Design review of the part built by this model. Coordinates are the model's own, in mm. Face numbers are marked on the shaded views. A direction names the side the tool comes from. Coordinates: 2 decimals unless noted, no trailing zeros. Loops run counter-clockwise (first coordinate to the right, second up) from the corner with the lowest first, then second, coordinate; pieces in that order, holes last. Notation, with made-up numbers: (-13.5, 72) -> (34.5, 72) arc R20 cw to (34.5, 87) -> close; hole circle Ø5 at (83.5, -38). An arc over 180 degrees is marked (long way). Use one line per item in the form item = value. Start each with the question number.
1. Consider section C-C (x = 21). State the section outline as (y, z) points.
2. The part is to be moulded in two halves that separate along X. For the marked faces 1, 2 and 3, say which applies: released by +X, released by -X, zero draft, split by the parting line, or undercut.
3. For pin 1 (5 mm diameter, centred on x = -25, z = 7, fed in from +Y); pin 2 (4 mm diameter, centred on x = 11.5, z = 1.5, fed in from -Y); pin 3 (2 mm diameter, centred on x = 5.5, z = 8.5, fed in from +Y), all flat-tipped, find the tip position at first contact; note any pin that passes through.
4. Machinability: for the marked faces 4, 5 and 6, which of the approach directions +Z, -Z, +X, -X, +Y, -Y give a long, thin tool a straight path to every point of the face, cutting with its end or side? Answer none if there is none.
5. Wall thickness on line 1 (X direction, y = 2.4, z = 5); line 2 (Y direction, x = 24.5, z = 2.75); line 3 (X direction, y = 1.2, z = 5): over which ranges is each line inside the solid? List them lowest first. Write a range as from..to.
6. Consider section A-A (z = 5). State the section outline as (x, y) points.
7. Consider section D-D (y = 13). State the section outline as (x, z) points, then the cut area to 3 significant figures.
8. Consider section B-B (y = 4.75). State the section outline as (x, z) points, then the cut area to 3 significant figures.
from build123d import *

# Parameters (mm, degrees)
BOSS_EXTRUDE1_DEPTH = 10
SKETCH2_R           = 1.5875
CUT_EXTRUDE1_DEPTH  = 3.765696


with BuildPart() as part:
    # Sketch1 → Boss-Extrude1 (new body)
    with BuildSketch(Plane.XY):
        with BuildLine():
            Line((-20, 0), (-15, 0))
            ThreePointArc((-15, 0), (0, 15), (15, 0))
            Line((15, 0), (20, 0))
            Line((20, 0), (30, 0))
            Line((30, 0), (30, 3.765695973))
            Line((30, 3.765695973), (19.642289425, 3.765695973))
            ThreePointArc((19.642289425, 3.765695973), (0, 20), (-19.642289425, 3.765695973))
            Line((-19.642289425, 3.765695973), (-30, 3.765695973))
            Line((-30, 3.765695973), (-30, 0))
            Line((-30, 0), (-20, 0))
        make_face()
    extrude(amount=BOSS_EXTRUDE1_DEPTH)

    # Sketch2 → Cut-Extrude1 (cut)
    with BuildSketch(Plane(origin=(0, 3.765695973, 0), x_dir=(1, 0, 0), z_dir=(0, 1, 0))):
        with Locations((24.821144712, -5)):
            Circle(SKETCH2_R)
    cut_extrude1 = extrude(amount=-CUT_EXTRUDE1_DEPTH, mode=Mode.SUBTRACT)

    # Mirror1: Cut-Extrude1 across plane
    add(cut_extrude1.mirror(Plane.ZY), mode=Mode.SUBTRACT)


solid = part.part
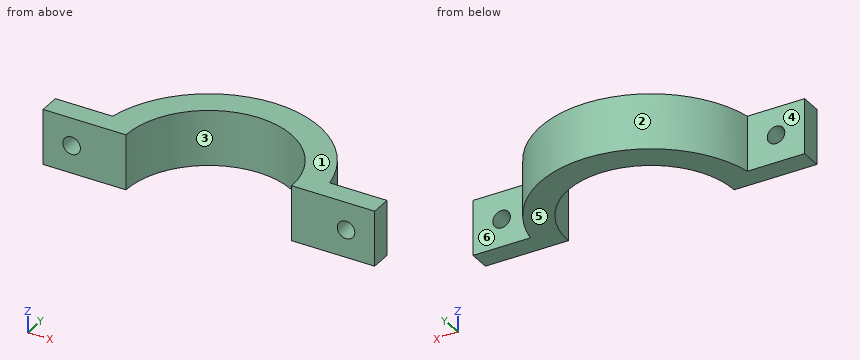
Geometry check:
q1.outline = (0, 0) -> (3.77, 0) -> (3.77, 10) -> (0, 10) -> close
q2.face_1 = zero draft
q2.face_2 = split by the parting line
q2.face_3 = undercut
q3.pin_1 = 3.77
q3.pin_2 = 6.54
q3.pin_3 = 19.49
q4.face_4 = +Z, -Z, -X, +Y
q4.face_5 = -Z, +X, -X, +Y, -Y
q4.face_6 = +Z, -Z, +X, +Y
q5.line_1 = -30..-26.41, -23.23..-14.81, 14.81..23.23, 26.41..30
q5.line_2 = 0..3.77
q5.line_3 = -30..-26.41, -23.23..-14.95, 14.95..23.23, 26.41..30
q6.outline = (-30, 0) -> (-26.41, 0) -> (-26.41, 3.77) -> (-30, 3.77) -> close; (-23.23, 0) -> (-15, 0) arc R15 cw to (15, 0) -> (23.23, 0) -> (23.23, 3.77) -> (19.64, 3.77) arc R20 ccw to (-19.64, 3.77) -> (-23.23, 3.77) -> close; (26.41, 0) -> (30, 0) -> (30, 3.77) -> (26.41, 3.77) -> close
q7.outline = (-15.2, 0) -> (-7.48, 0) -> (-7.48, 10) -> (-15.2, 10) -> close; (7.48, 0) -> (15.2, 0) -> (15.2, 10) -> (7.48, 10) -> close
q7.area = 154 mm²
q8.outline = (-19.43, 0) -> (-14.23, 0) -> (-14.23, 10) -> (-19.43, 10) -> close; (14.23, 0) -> (19.43, 0) -> (19.43, 10) -> (14.23, 10) -> close
q8.area = 104 mm²
